For this review, take the finished solid that the model builds, in its own axes (mm). Face numbers are marked on the shaded views. Coordinates: 2 decimals unless noted, no trailing zeros. Write each loop counter-clockwise with the first axis right and the second up, starting at its lowest first coordinate (ties: lowest second). Pieces come first, ordered by that corner, then holes. Notation, with made-up numbers: (10.5, 86) - (38.5, 86) arc R26 ccw to (38.5, 100) - close; hole circle Ø7 at (87.25, 34). An arc over 180 degrees is marked (long way). Write each question's results on one line, items separated by ' | '.
from build123d import *

# Parameters (mm, degrees)
SKETCH2_R           = 15
BOSS_EXTRUDE1_DEPTH = 9.8
CHAMFER1_SIZE       = 1
SHELL1_T            = -1
SKETCH7_W           = 2.5
SKETCH7_H           = 1
BOSS_EXTRUDE5_DEPTH = 1
CIRPATTERN1_COUNT   = 4


with BuildPart() as part:
    # Sketch1 → Revolve2 (revolve)
    with BuildSketch(Plane.XY):
        with BuildLine():
            Line((-25, 10), (-26.741669751, 3.5))
            Line((-26.741669751, 3.5), (-28.5, 3.5))
            Line((-28.5, 3.5), (-28.5, 2))
            Line((-28.5, 2), (-29.258330249, 2))
            Line((-29.258330249, 2), (-30, 0))
            Line((-30, 0), (-28.660254038, -5))
            Line((-28.660254038, -5), (-27.901923789, -5))
            Line((-27.901923789, -5), (-27.5, -6.5))
            ThreePointArc((-27.5, -6.5), (-24.083958056, -9.082951062), (-19.900657923, -10))
            Line((-19.900657923, -10), (0, -10))
            Line((0, -10), (0, 10))
            Line((0, 10), (-25, 10))
        make_face()
    revolve(axis=Axis((0, 614.019679743, 0), (0, -1, 0)))

    # Sketch2 → Boss-Extrude1 (add)
    with BuildSketch(Plane(origin=(0, 10, 0), x_dir=(1, 0, 0), z_dir=(0, 1, 0))):
        with Locations(Location((0, 0, 0), (0, 0, 180))):
            Circle(SKETCH2_R)
    extrude(amount=BOSS_EXTRUDE1_DEPTH)

    # Chamfer1
    chamfer1_edges = [part.edges().sort_by_distance(p)[0] for p in [
        (15, 19.8, 0),
    ]]
    chamfer(chamfer1_edges, length=CHAMFER1_SIZE)

    # Shell1
    shell1_openings = [part.faces().sort_by_distance(p)[0] for p in [
        (0, 19.8, 0),
    ]]
    offset(amount=SHELL1_T, openings=shell1_openings, kind=Kind.INTERSECTION)

    # Sketch7 → Boss-Extrude5 (add)
    with BuildSketch(Plane(origin=(0, 10, 0), x_dir=(1, 0, 0), z_dir=(0, 1, 0))):
        with Locations((-20.75, -0.5)):
            Rectangle(SKETCH7_W, SKETCH7_H)
    boss_extrude5 = extrude(amount=BOSS_EXTRUDE5_DEPTH)

    # CirPattern1: Boss-Extrude5 ×4 about axis
    cirpattern1_axis = Axis((0, 0, 0), (0, 1, 0))
    for i in range(1, CIRPATTERN1_COUNT):
        add(boss_extrude5.rotate(cirpattern1_axis, i * 360 / CIRPATTERN1_COUNT))


solid = part.part
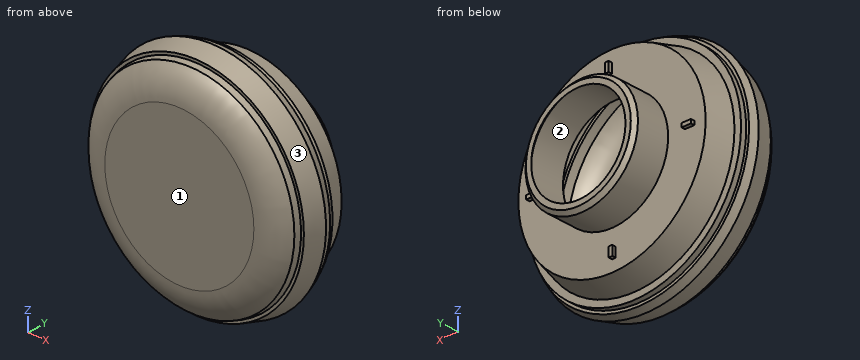
Q1. Mouldability with a two-part tool opening along X and no side actions: class the marked faces 1, 2 and 3 as pulls with the +X half, pulls with the -X half, needs draft (parallel to the pull), parting line crosses it, or undercut.
Results found:
face 1: needs draft | face 2: undercut | face 3: parting line crosses it
Q2. Take a section at A-A on y = 11.75. State the section outline as (x, z) points.
Results found:
outline: circle Ø30 at (0, 0); hole circle Ø28 at (0, 0)
Q3. Take a section at B-B on y = -2.25. State the section outline as (x, z) points.
Results found:
outline: circle Ø58.79 at (0, 0); hole circle Ø56.72 at (0, 0)
Q4. Wall thickness on line 1 along Y through (x, z) = (-12.5, -11); line 2 along Z through (x, y) = (0, 14.75); line 3 along Y through (x, z) = (10, -2): over which ranges is each line inside the solid? List them lowest first. Write a range as from..to.
Results found:
line 1: -10..-9, 9..10 | line 2: -15..-14, 14..15 | line 3: -10..-9
Q5. For pin 1 (5 mm diameter, centred on y = 9, z = -0.5, fed in from +X); pin 2 (0.8 mm diameter, centred on y = 10.5, z = 0.5, fed in from +X); pin 3 (4 mm diameter, centred on y = 16, z = 0, fed in from -X), all flat-tipped, find the tip position at first contact; note any pin that passes through.
Results found:
pin 1: x = 25.93 | pin 2: x = 15 | pin 3: x = -15
